Answer from the drawing. Dimensions are ordinates in mm from the lowest x, y and z of the part. Coordinates: 2 decimals unless noted, no trailing zeros. Write each loop counter-clockwise with the first axis right and the second up, starting at its lowest first coordinate (ties: lowest second). Pieces come first, ordered by that corner, then holes. Notation, with made-up numbers: (-28.5, 74.5) -> (-23.5, 74.5) arc R18 ccw to (-23.5, 102.5) -> close; hole circle Ø10 at (4.25, 76.5). An arc over 180 degrees is marked (long way). Return JSON: item names as keys, results as strings.
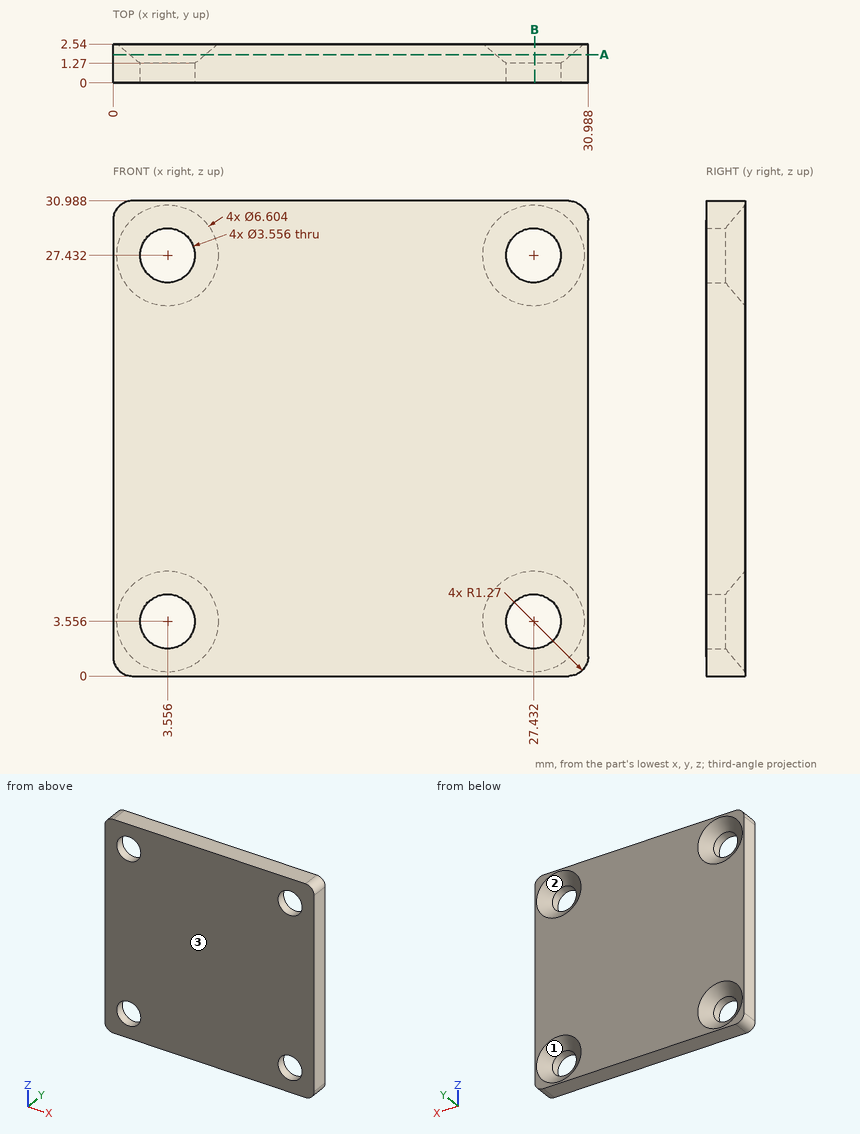
1. The part is cut by section B-B (x = 27.5). Count the separate pieces of the cut face and the enclosed holes in it, then the cut area to 3 significant figures.
Taken from the geometry:
{"separate pieces": "3", "enclosed holes": "0", "area": "56.8 mm2"}
2. For a pull along Z with two mould halves and no side action, classify the marked faces 1, 2 and 3 as +Z half, -Z half, draft (parallel to the pull), parting line (faces both ways), or undercut.
Taken from the geometry:
{"face 1": "undercut", "face 2": "undercut", "face 3": "draft"}
3. A flat-ended cylindrical pin translates along its axis: pin 1 Ø5.5 at (x, z) = (27.432, 3.556) entering from +Y. Find the tip coordinate at first contact, or state that the pin passes through.
Taken from the geometry:
{"pin 1": "stops at y = 2.08"}
4. The part is cut by section A-A (y = 1.85). Determine the outline of the cut face in (x, z), then the cut area to 3 significant figures.
Taken from the geometry:
{"outline": "(0, 1.27) arc R1.27 ccw to (1.27, 0) -> (29.72, 0) arc R1.27 ccw to (30.99, 1.27) -> (30.99, 29.72) arc R1.27 ccw to (29.72, 30.99) -> (1.27, 30.99) arc R1.27 ccw to (0, 29.72) -> close; hole circle Ø4.95 at (3.56, 3.56); hole circle Ø4.95 at (3.56, 27.43); hole circle Ø4.95 at (27.43, 3.56); hole circle Ø4.95 at (27.43, 27.43)", "area": "882 mm2"}
5. Consider L1, parallel to X at y = 0.7, z = 3.5; L2, parallel to Z at x = 28, y = 1.9; L3, parallel to X at y = 0.8, z = 29. Determine where each line is inside the solid, lowest interval first.
Taken from the geometry:
{"L1": "x = 0 to 1.78, 5.33 to 25.65, 29.21 to 30.99", "L2": "z = 0 to 1.09, 6.03 to 24.96, 29.9 to 30.99", "L3": "x = 0 to 2.72, 4.39 to 26.59, 28.27 to 30.99"}
